```python
from build123d import *

# Parameters (mm, degrees)
SKETCH1_R           = 30
BOSS_EXTRUDE1_DEPTH = 5
SKETCH2_R           = 5
CUT_EXTRUDE1_DEPTH  = 5
SKETCH3_R           = 15
BOSS_EXTRUDE2_DEPTH = 35
SKETCH4_R           = 7.5
CUT_EXTRUDE2_DEPTH  = 68.268120235


with BuildPart() as part:
    # Sketch1 → Boss-Extrude1 (new body)
    with BuildSketch(Plane(origin=(0, 0, 0), x_dir=(1, 0, 0), z_dir=(0, 1, 0))):
        with Locations(Location((0, 0, 0), (0, 0, 270))):
            Circle(SKETCH1_R)
    extrude(amount=BOSS_EXTRUDE1_DEPTH)

    # Sketch2 → Cut-Extrude1 (cut)
    with BuildSketch(Plane(origin=(0, 5, 0), x_dir=(1, 0, 0), z_dir=(0, 1, 0))):
        with Locations(Location((0, 22.5, 0), (0, 0, 270))):
            Circle(SKETCH2_R)
        with Locations(Location((22.5, 0, 0), (0, 0, 270))):
            Circle(SKETCH2_R)
        with Locations(Location((0, -22.5, 0), (0, 0, 270))):
            Circle(SKETCH2_R)
        with Locations(Location((-22.5, 0, 0), (0, 0, 270))):
            Circle(SKETCH2_R)
    extrude(amount=-CUT_EXTRUDE1_DEPTH, mode=Mode.SUBTRACT)

    # Sketch3 → Boss-Extrude2 (add)
    with BuildSketch(Plane(origin=(0, 5, 0), x_dir=(1, 0, 0), z_dir=(0, 1, 0))):
        with Locations(Location((0, 0, 0), (0, 0, 270))):
            Circle(SKETCH3_R)
    extrude(amount=BOSS_EXTRUDE2_DEPTH)

    # Sketch4 → Cut-Extrude2 (cut, through all)
    with BuildSketch(Plane.XY.offset(15)):
        with Locations(Location((0, 25, 0), (0, 0, 90.000000014))):
            Circle(SKETCH4_R)
    extrude(amount=-CUT_EXTRUDE2_DEPTH, mode=Mode.SUBTRACT)


solid = part.part
```
Geometry check sheet. Reference: the model listing, model coordinates, mm. A direction names the side the tool comes from. Give positions to 0.01 mm unless a question says otherwise; leave off trailing zeros. Loops run counter-clockwise (first coordinate to the right, second up) from the corner with the lowest first, then second, coordinate; pieces in that order, holes last. Notation, with made-up numbers: M -16,13.25 L 39,13.25 A21 ccw 39,52.25 Z; hole C 79.5,63.5 d6. An arc over 180 degrees is marked long. Write item = value, one per line.
(1) Gauge pin test, flat ends, axial feed: pin 1 Ø5 at (y, z) = (19, 2.5) entering from +X; pin 2 Ø10 at (x, z) = (3, 21) entering from -Y; pin 3 Ø10 at (y, z) = (23.5, 14.5) entering from +X; pin 4 Ø3 at (x, z) = (-10.5, 15) entering from +Y. Record the tip position at first contact, or that the pin passes through.
Answer below:
pin_1 = 15
pin_2 = 0
pin_3 = 11.61
pin_4 = 5
(2) Sectioned sample at B-B, the plane x = 0. Record the cut outline in (y, z), plus the area to 3 significant figures.
Answer below:
outline = M 0,-30 L 5,-30 L 5,-27.5 L 0,-27.5 Z; M 0,-17.5 L 5,-17.5 L 5,-15 L 17.5,-15 L 17.5,15 L 5,15 L 5,17.5 L 0,17.5 Z; M 0,27.5 L 5,27.5 L 5,30 L 0,30 Z; M 32.5,-15 L 40,-15 L 40,15 L 32.5,15 Z
area = 800 mm2
(3) Sectioned sample at D-D, the plane x = -22.5. Record the cut outline in (y, z), plus the area to 3 significant figures.
Answer below:
outline = M 0,-19.84 L 5,-19.84 L 5,-5 L 0,-5 Z; M 0,5 L 5,5 L 5,19.84 L 0,19.84 Z
area = 148 mm2
(4) Sectioned sample at A-A, the plane z = 0. Record the cut outline in (x, y), plus the area to 3 significant figures.
Answer below:
outline = M -30,0 L -27.5,0 L -27.5,5 L -30,5 Z; M -17.5,0 L 17.5,0 L 17.5,5 L 15,5 L 15,40 L -15,40 L -15,5 L -17.5,5 Z; M 27.5,0 L 30,0 L 30,5 L 27.5,5 Z; hole C 0,25 d15
area = 1,070 mm2
(5) Release check for a two-part mould opening along Z. For faces 1 (the face through (-27.38, 2.54, -1.08)), 2 (the face through (-9, 22, -12)), 3 (the face through (-6.324, 29.032, 0.21)) record: released by +Z, released by -Z, zero draft, split by the parting line, or undercut.
Answer below:
face_1 = undercut
face_2 = split by the parting line
face_3 = zero draft
(6) Sectioned sample at C-C, the plane z = 22.5. Record the cut outline in (x, y), plus the area to 3 significant figures.
Answer below:
outline = M -19.84,0 L -5,0 L -5,5 L -19.84,5 Z; M 5,0 L 19.84,0 L 19.84,5 L 5,5 Z
area = 148 mm2
(7) Tool access check on faces 4 (the face through (14, 5, 6)), 5 (the face through (1.32, 2.46, -29.97)). Record the directions out of +Z, -Z, +X, -X, +Y, -Y that give a thin tool (end or side, any length) a straight path to the whole face; none if there is none.
Answer below:
face_4 = +Y
face_5 = +Y, -Y
(8) Material ranges on line 1 (X direction, y = 2.7, z = 0); line 2 (Y direction, x = 0, z = 10); line 3 (X direction, y = 2.5, z = -1), recorded low to high. Write a range as [from, to].
Answer below:
line_1 = [-30, -27.5], [-17.5, 17.5], [27.5, 30]
line_2 = [0, 17.5], [32.5, 40]
line_3 = [-29.98, -27.4], [-17.6, 17.6], [27.4, 29.98]
